Verification items for the finished model (mm, model axes). A direction names the side the tool comes from. Round coordinates to 2 decimals unless told otherwise and drop trailing zeros. Write each loop counter-clockwise with the first axis right and the second up, starting at its lowest first coordinate (ties: lowest second). Pieces come first, ordered by that corner, then holes. Notation, with made-up numbers: M 84.25,79 L 98.25,79 A17 cw 98.25,107 Z; hole C -13.75,77.25 d1. An arc over 180 degrees is marked long. One line per question, with ' | ' between items. Start each with the question number.
Q1. Tool access check on faces 1 (the face through (-14.56, -8.06, -12.65)), 2 (the face through (-133.26, 14.38, -0.9)). Record the directions out of +Z, -Z, +X, -X, +Y, -Y that give a thin tool (end or side, any length) a straight path to the whole face; none if there is none.
Q2. Gauge pin test, flat ends, axial feed: pin 1 (11 mm diameter, centred on y = 0, z = 0, fed in from -X); pin 2 (10 mm diameter, centred on x = 82.5, y = -7.5, fed in from +Z); pin 3 (1.5 mm diameter, centred on x = 73, z = -10, fed in from +Y); pin 4 (2 mm diameter, centred on x = 52, y = 1.5, fed in from +Z). Record the tip position at first contact, or that the pin passes through.
Q3. Thickness scan on line 1 along Z through (x, y) = (132, 0); line 2 along X through (y, z) = (-12.5, -8); line 3 along Z through (x, y) = (-31, 4.5). Record the ranges inside material, lowest first. Write a range as from..to.
Q4. Cross-section at A-A (x = 86.5). Record the boundary of the cut face in (y, z).
Q5. Release check for a two-part mould opening along X. For faces 3 (the face through (119.79, 1.86, -14.18)), 4 (the face through (-23.21, 1.86, -14.18)), 5 (the face through (113.562, -0.576, 0.128)), 6 (the face through (139.28, -8.06, -12.65)) record: released by +X, released by -X, zero draft, split by the parting line, or undercut.
from build123d import *

# Parameters (mm, degrees)
M8_GEWINDEBOHRUNG1_D               = 6.8
M8_GEWINDEBOHRUNG1_DEPTH           = 26.25
M8_GEWINDEBOHRUNG1_CSINK_D         = 8.1
M8_GEWINDEBOHRUNG1_CSINK_ANGLE     = 90
M8_GEWINDEBOHRUNG1_TIP             = 2.042926105
M8_GEWINDEBOHRUNG2_D               = 6.8
M8_GEWINDEBOHRUNG2_DEPTH           = 26.25
M8_GEWINDEBOHRUNG2_CSINK_D         = 8.1
M8_GEWINDEBOHRUNG2_CSINK_ANGLE     = 90
M8_GEWINDEBOHRUNG2_TIP             = 2.042926105
F_6_0_6_DURCHMESSER_BOHRUNG1_D     = 6
F_6_0_6_DURCHMESSER_BOHRUNG1_DEPTH = 1
F_6_0_6_DURCHMESSER_BOHRUNG1_TIP   = 1.802581857


with BuildPart() as part:
    # Skizze1 → Basis-Rotation (revolve)
    with BuildSketch(Plane.XY, mode=Mode.PRIVATE) as basis_rotation_sk:
        Polygon((-141.5, 14), (-141.5, 0), (141.5, 0), (141.5, 14), (140.5, 15), (138.1, 15), (138.1, 14.3), (136.5, 14.3), (136.5, 15), (120.6, 15), (120.6, 14.3), (119, 14.3), (119, 15), (-4.9, 15), (-4.9, 14.3), (-6.5, 14.3), (-6.5, 15), (-22.4, 15), (-22.4, 14.3), (-24, 14.3), (-24, 15), (-140.5, 15), align=None)
    revolve(basis_rotation_sk.sketch.rotate(Axis((-241.855208518, 0, 0), (1, 0, 0)), 180), axis=Axis((-241.855208518, 0, 0), (1, 0, 0)))

    # M8 Gewindebohrung1
    with Locations(Plane.ZY.offset(141.5)):
        with Locations((0, 0)):
            CounterSinkHole(M8_GEWINDEBOHRUNG1_D / 2, M8_GEWINDEBOHRUNG1_CSINK_D / 2, depth=M8_GEWINDEBOHRUNG1_DEPTH, counter_sink_angle=M8_GEWINDEBOHRUNG1_CSINK_ANGLE)
            with Locations((0, 0, -(M8_GEWINDEBOHRUNG1_DEPTH + M8_GEWINDEBOHRUNG1_TIP / 2))):  # 118° drill point
                Cone(0, M8_GEWINDEBOHRUNG1_D / 2, M8_GEWINDEBOHRUNG1_TIP, mode=Mode.SUBTRACT)

    # M8 Gewindebohrung2
    with Locations(Plane(origin=(141.5, 0, 0), x_dir=(0, 0, -1), z_dir=(1, 0, 0))):
        with Locations((0, 0)):
            CounterSinkHole(M8_GEWINDEBOHRUNG2_D / 2, M8_GEWINDEBOHRUNG2_CSINK_D / 2, depth=M8_GEWINDEBOHRUNG2_DEPTH, counter_sink_angle=M8_GEWINDEBOHRUNG2_CSINK_ANGLE)
            with Locations((0, 0, -(M8_GEWINDEBOHRUNG2_DEPTH + M8_GEWINDEBOHRUNG2_TIP / 2))):  # 118° drill point
                Cone(0, M8_GEWINDEBOHRUNG2_D / 2, M8_GEWINDEBOHRUNG2_TIP, mode=Mode.SUBTRACT)

    # 6.0 _6_ Durchmesser Bohrung1
    with Locations(Plane(origin=(0, 15, 0), x_dir=(1, 0, 0), z_dir=(0, 1, 0))):
        with Locations((-50.4, 0), (-130.4, 0)):
            Hole(F_6_0_6_DURCHMESSER_BOHRUNG1_D / 2, depth=F_6_0_6_DURCHMESSER_BOHRUNG1_DEPTH)
            with Locations((0, 0, -(F_6_0_6_DURCHMESSER_BOHRUNG1_DEPTH + F_6_0_6_DURCHMESSER_BOHRUNG1_TIP / 2))):  # 118° drill point
                Cone(0, F_6_0_6_DURCHMESSER_BOHRUNG1_D / 2, F_6_0_6_DURCHMESSER_BOHRUNG1_TIP, mode=Mode.SUBTRACT)


solid = part.part
Determined:
1) face 1: +X, -X | face 2: +Y
2) pin 1: stops at x = -141.5 | pin 2: stops at z = 14.79 | pin 3: stops at y = 11.81 | pin 4: stops at z = 14.99
3) line 1: z = -15..-3.4, 3.4..15 | line 2: x = -140.66..-24, -22.4..-6.5, -4.9..119, 120.6..136.5, 138.1..140.66 | line 3: z = -14.31..14.31
4) outline: C 0,0 d30
5) face 3: undercut | face 4: undercut | face 5: released by +X | face 6: zero draft
